Model file for the job. Use its own axes, mm. A direction names the side the tool comes from. Round coordinates to 2 decimals unless told otherwise and drop trailing zeros. Order: outer loops, then holes, each group sorted by start corner. A loop starts at its lowest first (then second) coordinate and runs counter-clockwise, first axis right, second up. Notation, with made-up numbers: M 62,-5.5 L 113,-5.5 A21 cw 113,20.5 Z; hole C 7,49 d10. An arc over 180 degrees is marked long. Return JSON: item names as keys, results as strings. Group by question number.
Item 1: Slice it at D-D on z = 8. Write the cut outline in (x, y), then the cut area to 3 significant figures.
Item 2: Pull direction X, two halves, no side cores. Call faces 1 (the face through (1.79, 0.03, -19.51)), 2 (the face through (-2.16, 0.48, -19.51)), 3 (the face through (-2, 0, -32.385)), 4 (the face through (1.699, -3.267, -3.444)): pulls with the +X half, pulls with the -X half, needs draft (parallel to the pull), parting line crosses it, or undercut.
Item 3: Slice it at C-C on x = -1.25. Write the cut outline in (y, z) (3 decimals), then the cut area to 3 significant figures.
Item 4: Which spindle directions (+Z, -Z, +X, -X, +Y, -Y) get a long thin tool onto all of the face, cutting with end or side? Do faces 5 (the face through (-0.488, 3.715, 9.392)), 6 (the face through (0, 0, -6.985)). Say none if no direction does.
Item 5: Probe line 1 along Z through (x, y) = (1.75, -2) (3 decimals); line 2 along Y through (x, z) = (-0.25, 2.5); line 3 along Y through (x, z) = (-1.5, -11.5). List the from-to ranges inside material, lowest first.
Item 6: Pin check, flat tips, straight feed: pin 1 Ø1.5 at (x, z) = (1, -24.5) entering from -Y; pin 2 Ø3 at (x, z) = (1.5, -8) entering from +Y. Stop position of each tip, or through.
Item 7: Slice it at B-B on z = -8.5. Write the cut outline in (x, y).
from build123d import *

# Parameters (mm, degrees)
F0_R     = 3.683
F1_DEPTH = 6.985
F2_R     = 0.7874
F3_DEPTH = 25.4
F4_R     = 3.7465
F5_DEPTH = 19.05


with BuildPart() as f1:
    # F0 (on Top) → F1 (new body)
    with BuildSketch(Plane.XY):
        Circle(F0_R)
    extrude(amount=-F1_DEPTH)

    # F2 (on face) → F3 (join)
    with BuildSketch(Plane(origin=(0, 0, -6.985), x_dir=(1, 0, 0), z_dir=(0, 0, -1))):
        with BuildLine():
            ThreePointArc((1.7907, 0), (1.0033, 0.7874), (0.2159, 0))
            ThreePointArc((0.2159, 0), (1.0033, -0.7874), (1.7907, 0))
        make_face()
        with Locations((-1.5367, 0)):
            Circle(F2_R)
    extrude(amount=F3_DEPTH)

    # F4 (on face) → F5 (join)
    with BuildSketch(Plane.XY):
        Circle(F4_R)
    extrude(amount=F5_DEPTH)


solid = f1.part
Output values:
{
 "1": {"outline": "C 0,0 d7.49", "area": "44.1 mm²"},
 "2": {"face 1": "undercut", "face 2": "undercut", "face 3": "needs draft", "face 4": "parting line crosses it"},
 "3": {"outline": "M -3.532,0 L -3.464,0 L -3.464,-6.985 L -0.733,-6.985 L -0.733,-32.385 L 0.733,-32.385 L 0.733,-6.985 L 3.464,-6.985 L 3.464,0 L 3.532,0 L 3.532,19.05 L -3.532,19.05 Z", "area": "220 mm²"},
 "4": {"face 5": "+Z, -Z", "face 6": "-Z"},
 "5": {"line 1": "-6.985 to 19.05", "line 2": "-3.74 to 3.74", "line 3": "-0.79 to 0.79"},
 "6": {"pin 1": "y = -0.79", "pin 2": "y = 3.66"},
 "7": {"outline": "C -1.54,0 d1.57; C 1,0 d1.57"}
}
